from build123d import *

# Parameters (mm, degrees)
SKETCH_1_W          = 300
SKETCH_1_H          = 150
EXTRUDE_1_DEPTH     = 30
SKETCH_2_R          = 15
EXTRUDE_2_DEPTH     = 50
SKETCH_3_R          = 30
CUT_EXTRUDE_1_DEPTH = 50


with BuildPart() as part:
    # 草图1 → 凸台-拉伸1 (new body)
    with BuildSketch(Plane(origin=(0, 0, 0), x_dir=(1, 0, 0), z_dir=(0, 1, 0))):
        Rectangle(SKETCH_1_W, SKETCH_1_H)
    extrude(amount=EXTRUDE_1_DEPTH)

    # 草图2 → 凸台-拉伸2 (add)
    with BuildSketch(Plane(origin=(0, 30, 0), x_dir=(1, 0, 0), z_dir=(0, 1, 0))):
        with Locations((-100, 0)):
            Circle(SKETCH_2_R)
        with Locations((100, 0)):
            Circle(SKETCH_2_R)
    extrude(amount=EXTRUDE_2_DEPTH)

    # 草图3 → 切除-拉伸1 (cut)
    with BuildSketch(Plane(origin=(0, 30, 0), x_dir=(1, 0, 0), z_dir=(0, 1, 0))):
        Circle(SKETCH_3_R)
    extrude(amount=-CUT_EXTRUDE_1_DEPTH, mode=Mode.SUBTRACT)


solid = part.part
Geometry: final body of the model. Coordinates: model frame, mm. A direction names the side the tool comes from. Give positions to 0.01 mm unless a question says otherwise; leave off trailing zeros. Order: outer loops, then holes, each group sorted by start corner. A loop starts at its lowest first (then second) coordinate and runs counter-clockwise, first axis right, second up. Notation, with made-up numbers: (-18, 68) -> (26, 68) arc R18 cw to (26, 79) -> close; hole circle Ø10 at (52.5, 75). An arc over 180 degrees is marked (long way). Put each result on its own line as item: value.
Q1. Section B-B, the plane x = 0. Return loops of the section in (y, z).
Here are the results:
outline: (0, -75) -> (30, -75) -> (30, -30) -> (0, -30) -> close; (0, 30) -> (30, 30) -> (30, 75) -> (0, 75) -> close
Q2. Section A-A, the plane z = 0. Return loops of the section in (x, y), then the cut area to 3 significant figures.
Here are the results:
outline: (-150, 0) -> (-30, 0) -> (-30, 30) -> (-85, 30) -> (-85, 80) -> (-115, 80) -> (-115, 30) -> (-150, 30) -> close; (30, 0) -> (150, 0) -> (150, 30) -> (115, 30) -> (115, 80) -> (85, 80) -> (85, 30) -> (30, 30) -> close
area: 10,200 mm^2
Q3. Section D-D, the plane y = 66.5. Return loops of the section in (x, z).
Here are the results:
outline: circle Ø30 at (-100, 0); circle Ø30 at (100, 0)
Q4. Draft query along X for faces 3 (the face through (100, 80, 0)), 4 (the face through (-29.97, 15.21, -1.32)), 5 (the face through (150, 15, 1)). Return one class per face: released by +X, released by -X, zero draft, split by the parting line, or undercut.
Here are the results:
face 3: zero draft
face 4: undercut
face 5: released by +X
Q5. Section C-C, the plane y = 25.5. Return loops of the section in (x, z), then the cut area to 3 significant figures.
Here are the results:
outline: (-150, -75) -> (150, -75) -> (150, 75) -> (-150, 75) -> close; hole circle Ø60 at (0, 0)
area: 42,200 mm^2
Q6. Reachability of faces 1 (the face through (-85.693, 54.65, -4.506)), 2 (the face through (-2, 15, 75)) from +Z, -Z, +X, -X, +Y, -Y: full face, straight path, thin tool, end or side. Return the list, or none.
Here are the results:
face 1: +Y
face 2: +Z, +X, -X, +Y, -Y
Q7. Material intervals for L1, parallel to Z at x = 0, y = 9; L2, parallel to X at y = 24.25, z = 0; L3, parallel to Y at x = 94, z = 17, sorted ascending.
Here are the results:
L1: z = -75 to -30, 30 to 75
L2: x = -150 to -30, 30 to 150
L3: y = 0 to 30
Q8. Pin query (flat end, axial travel): pin 1 (4 mm diameter, centred on y = 45.5, z = 14.5, fed in from -X); pin 2 (4 mm diameter, centred on x = -85, z = -38, fed in from +Y); pin 3 (12 mm diameter, centred on x = -115.5, y = 70.5, fed in from -Z). Return the tip coordinate at first contact, or that it passes through.
Here are the results:
pin 1: stops at x = -108.29
pin 2: stops at y = 30
pin 3: stops at z = -11.61
